from build123d import *

# Parameters (mm, degrees)
SKETCH1_W           = 100
SKETCH1_H           = 100
BOSS_EXTRUDE1_DEPTH = 4
SKETCH2_R           = 4.75
CUT_EXTRUDE1_DEPTH  = 2
SKETCH3_R           = 5.5
CUT_EXTRUDE2_DEPTH  = 5


with BuildPart() as part:
    # Sketch1 → Boss-Extrude1 (new body)
    with BuildSketch(Plane.XY):
        Rectangle(SKETCH1_W, SKETCH1_H)
    extrude(amount=BOSS_EXTRUDE1_DEPTH)

    # Sketch2 → Cut-Extrude1 (cut)
    with BuildSketch(Plane(origin=(0, 0, 0), x_dir=(-1, 0, 0), z_dir=(0, 0, -1))):
        with Locations((45, 45)):
            Circle(SKETCH2_R)
        with Locations((45, -45)):
            Circle(SKETCH2_R)
        with Locations((-45, -45)):
            Circle(SKETCH2_R)
        with Locations((-45, 45)):
            Circle(SKETCH2_R)
    extrude(amount=-CUT_EXTRUDE1_DEPTH, mode=Mode.SUBTRACT)

    # Sketch3 → Cut-Extrude2 (cut, through all)
    with BuildSketch(Plane(origin=(-38.404344239, -79.614153906, 4), x_dir=(1, 0, 0), z_dir=(0, 0, 1))):
        with Locations((58.387586461, 99.345162416)):
            Circle(SKETCH3_R)
    extrude(amount=-CUT_EXTRUDE2_DEPTH, mode=Mode.SUBTRACT)


solid = part.part
Geometry check sheet. Reference: the model listing, model coordinates, mm. A direction names the side the tool comes from. Give positions to 0.01 mm unless a question says otherwise; leave off trailing zeros. Order: outer loops, then holes, each group sorted by start corner. A loop starts at its lowest first (then second) coordinate and runs counter-clockwise, first axis right, second up.
1) Gauge pin test, flat ends, axial feed: pin 1 (3 mm diameter, centred on x = 43.5, y = 43.5, fed in from -Z); pin 2 (10.5 mm diameter, centred on x = -45.5, y = -43.5, fed in from -Z). Record the tip position at first contact, or that the pin passes through.
Results are:
pin 1: stops at z = 2
pin 2: stops at z = 0
2) Cross-section at A-A (x = 45). Record the boundary of the cut face in (y, z), then the cut area to 3 significant figures.
Results are:
outline: (-50, 0) - (-49.75, 0) - (-49.75, 2) - (-40.25, 2) - (-40.25, 0) - (40.25, 0) - (40.25, 2) - (49.75, 2) - (49.75, 0) - (50, 0) - (50, 4) - (-50, 4) - close
area: 362 mm2
3) Material ranges on probe 1 along Y at (x, z) = (-45, 1.05); probe 2 along Y at (x, z) = (19.5, 2.3); probe 3 along Y at (x, z) = (22.5, 0.3), recorded low to high.
Results are:
probe 1: y = -50 to -49.75, -40.25 to 40.25, 49.75 to 50
probe 2: y = -50 to 14.25, 25.21 to 50
probe 3: y = -50 to 14.84, 24.62 to 50
4) Cross-section at C-C (z = 1). Record the boundary of the cut face in (x, y), then the cut area to 3 significant figures.
Results are:
outline: (-50, -50) - (50, -50) - (50, 50) - (-50, 50) - close; hole circle Ø9.5 at (-45, -45); hole circle Ø9.5 at (-45, 45); hole circle Ø11 at (19.98, 19.73); hole circle Ø9.5 at (45, -45); hole circle Ø9.5 at (45, 45)
area: 9,620 mm2
5) Draft check along Y on faces 3 (the flat face through (-1, 50, 2)), 4 (the flat face through (-1, -50, 2)), 5 (the flat face through (-45, 45, 2)). Enter one of: released by +Y, released by -Y, zero draft, split by the parting line, or undercut.
Results are:
face 3: released by +Y
face 4: released by -Y
face 5: undercut
6) Cross-section at B-B (y = 16). Record the boundary of the cut face in (x, z), then the cut area to 3 significant figures.
Results are:
outline: (-50, 0) - (15.94, 0) - (15.94, 4) - (-50, 4) - close; (24.02, 0) - (50, 0) - (50, 4) - (24.02, 4) - close
area: 368 mm2
7) Tool access check on faces 1 (the cylindrical face through (-44.38, 49.71, 0.99)), 2 (the flat face through (-1, 1, 0)). Record the directions out of +Z, -Z, +X, -X, +Y, -Y that give a thin tool (end or side, any length) a straight path to the whole face; none if there is none.
Results are:
face 1: -Z
face 2: -Z, +X, -X, +Y, -Y
